Here's how the part is built. I have some questions about the finished solid (model axes, mm). Face numbers are marked on the shaded views. A direction names the side the tool comes from. Give positions to 0.01 mm unless a question says otherwise; leave off trailing zeros. Loops run counter-clockwise (first coordinate to the right, second up) from the corner with the lowest first, then second, coordinate; pieces in that order, holes last. Notation, with made-up numbers: M -36,33 L 20,33 A22 cw 20,62 Z; hole C -35.5,31.25 d8. An arc over 180 degrees is marked long. Answer as CSV lines item,"result". Start each with the question number.
Item 1: If I drill on line 1 along X through (y, z) = (3.5, 63.5) (3 decimals); line 2 along Z through (x, y) = (266.7, 11.25) (3 decimals); line 3 along X through (y, z) = (10, 56.5), over which ranges is the centre line in solid material (lowest first)? Write a range as from..to.
Item 2: I want a section at C-C on z = 88.5. List the corners of the cut face in (x, y) for me, plus the area to 3 significant figures.
Item 3: I want a section at A-A on z = 63.5. List the corners of the cut face in (x, y) for me (3 decimals).
Item 4: I want a section at B-B on x = 43.5. List the corners of the cut face in (y, z) for me, plus the area to 3 significant figures.
Item 5: Will these pins go through, and if not, where does the flat tip stop? P1, Ø1.5, axis at y = 17, z = 107, coming from the +X side; P2, Ø4, axis at y = 17.5, z = 23, coming from the -X side.
Item 6: For the marked faces 1, 2 and 3, which set-ups out of +Z, -Z, +X, -X, +Y, -Y let a thin tool reach every point of the face, with its end or its side?
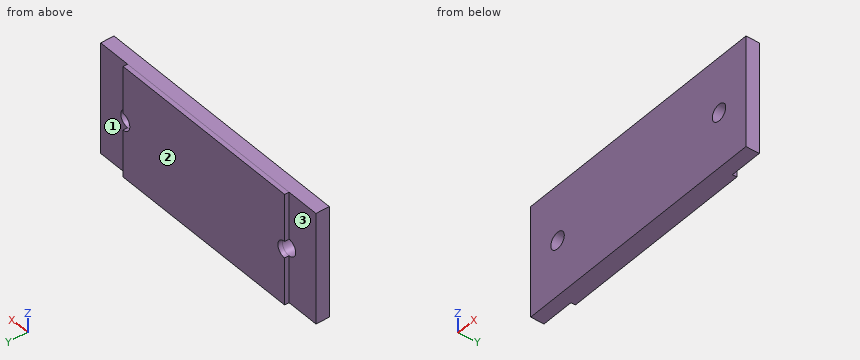
from build123d import *

# Parameters (mm, degrees)
SKETCH2_W           = 304.8
SKETCH2_H           = 127
SKETCH2_R           = 9.525
BOSS_EXTRUDE1_DEPTH = 15.24
BOSS_EXTRUDE2_DEPTH = 5.08


with BuildPart() as part:
    # Sketch2 → Boss-Extrude1 (new body)
    with BuildSketch(Plane(origin=(0, 0, 0), x_dir=(1, 0, 0), z_dir=(0, 1, 0))):
        with Locations((152.4, -63.5)):
            Rectangle(SKETCH2_W, SKETCH2_H)
        with Locations(Location((38.1, -63.5, 0), (0, 0, 90))):
            Circle(SKETCH2_R, mode=Mode.SUBTRACT)
        with Locations(Location((266.7, -63.5, 0), (0, 0, 90))):
            Circle(SKETCH2_R, mode=Mode.SUBTRACT)
    extrude(amount=BOSS_EXTRUDE1_DEPTH)

    # Sketch3 → Boss-Extrude2 (add)
    with BuildSketch(Plane(origin=(0, 15.24, 0), x_dir=(1, 0, 0), z_dir=(0, 1, 0))):
        with BuildLine():
            Line((38.1, 0), (266.7, 0))
            Line((266.7, 0), (266.7, -53.975))
            ThreePointArc((266.7, -53.975), (257.175, -63.5), (266.7, -73.025))
            Line((266.7, -73.025), (266.7, -127))
            Line((266.7, -127), (38.1, -127))
            Line((38.1, -127), (38.1, -73.025))
            ThreePointArc((38.1, -73.025), (47.625, -63.5), (38.1, -53.975))
            Line((38.1, -53.975), (38.1, 0))
        make_face()
    extrude(amount=BOSS_EXTRUDE2_DEPTH)


solid = part.part
Result:
1,line 1,"0..28.575, 47.625..257.175, 276.225..304.8"
1,line 2,"0..53.975, 73.025..127"
1,line 3,"0..31.64, 44.56..260.24, 273.16..304.8"
2,outline,"M 0,0 L 304.8,0 L 304.8,15.24 L 266.7,15.24 L 266.7,20.32 L 38.1,20.32 L 38.1,15.24 L 0,15.24 Z"
2,area,"5,810 mm^2"
3,outline,"M 0,0 L 28.575,0 L 28.575,15.24 L 0,15.24 Z; M 47.625,0 L 257.175,0 L 257.175,20.32 L 47.625,20.32 Z; M 276.225,0 L 304.8,0 L 304.8,15.24 L 276.225,15.24 Z"
4,outline,"M 0,0 L 20.32,0 L 20.32,55.65 L 0,55.65 Z; M 0,71.35 L 20.32,71.35 L 20.32,127 L 0,127 Z"
4,area,"2,260 mm^2"
5,P1,"x = 266.7"
5,P2,"x = 38.1"
6,face 1,"+Z, -Z, +X, +Y"
6,face 2,"+Z, -Z, +X, -X, +Y"
6,face 3,"+Z, -Z, -X, +Y"
